Work out the finished part from the listing and answer in its coordinate system (mm). Face numbers are marked on the shaded views. A direction names the side the tool comes from. Coordinates: 2 decimals unless noted, no trailing zeros. Order: outer loops, then holes, each group sorted by start corner. A loop starts at its lowest first (then second) coordinate and runs counter-clockwise, first axis right, second up. Notation, with made-up numbers: (3.5, 0) -> (8.5, 0) arc R15 cw to (8.5, 27) -> close; hole circle Ø7 at (13.5, 57.5). An arc over 180 degrees is marked (long way). Use one line per item in the form item = value.
from build123d import *

# Parameters (mm, degrees)
F1_DEPTH = 20
F2_R     = 2.25
F3_DEPTH = 25
F6_DEPTH = 200
F8_DEPTH = 25


with BuildPart() as f1:
    # F0 (on Top) → F1 (new body)
    with BuildSketch(Plane.XY):
        with BuildLine():
            Line((-14.1666658925, 2), (-14.1666658925, 0.5))
            ThreePointArc((-14.1666658925, 0.5), (-14.0202192831, 0.1464466094), (-13.6666658925, 0))
            Line((-13.6666658925, 0), (55.3333341075, 0))
            ThreePointArc((55.3333341075, 0), (55.6868874981, 0.1464466094), (55.8333341075, 0.5))
            Line((55.8333341075, 0.5), (55.8333341075, 2))
            ThreePointArc((55.8333341075, 2), (55.6868874981, 2.3535533906), (55.3333341075, 2.5))
            Line((55.3333341075, 2.5), (42.8333341075, 2.5))
            ThreePointArc((42.8333341075, 2.5), (41.4191205451, 3.0857864376), (40.8333341075, 4.5))
            Line((40.8333341075, 4.5), (40.8333341075, 5))
            ThreePointArc((40.8333341075, 5), (39.3688680134, 8.5355339059), (35.8333341075, 10))
            Line((35.8333341075, 10), (5.8333341075, 10))
            ThreePointArc((5.8333341075, 10), (2.2978002016, 8.5355339059), (0.8333341075, 5))
            Line((0.8333341075, 5), (0.8333341075, 4.5))
            ThreePointArc((0.8333341075, 4.5), (0.2475476699, 3.0857864376), (-1.1666658925, 2.5))
            Line((-1.1666658925, 2.5), (-13.6666658925, 2.5))
            ThreePointArc((-13.6666658925, 2.5), (-14.0202192831, 2.3535533906), (-14.1666658925, 2))
        make_face()
        Polygon((3.2352578961, 6.25), (4.5342960018, 8.5), (7.1323722132, 8.5), (8.4314103188, 6.25), (7.1323722132, 4), (4.5342960018, 4), align=None, mode=Mode.SUBTRACT)
        Polygon((11.3126081653, 6.25), (12.3229711364, 8), (14.3436970786, 8), (15.3540600497, 6.25), (14.3436970786, 4.5), (12.3229711364, 4.5), align=None, mode=Mode.SUBTRACT)
        Polygon((19.1012832999, 6.25), (19.9673087037, 7.75), (21.6993595113, 7.75), (22.5653849151, 6.25), (21.6993595113, 4.75), (19.9673087037, 4.75), align=None, mode=Mode.SUBTRACT)
        Polygon((26.8899584345, 6.25), (27.611646271, 7.5), (29.055021944, 7.5), (29.7767097805, 6.25), (29.055021944, 5), (27.611646271, 5), align=None, mode=Mode.SUBTRACT)
        Polygon((34.6786335691, 6.25), (35.2559838383, 7.25), (36.4106843767, 7.25), (36.9880346459, 6.25), (36.4106843767, 5.25), (35.2559838383, 5.25), align=None, mode=Mode.SUBTRACT)
    extrude(amount=F1_DEPTH)

    # F2 (on face) → F3 (cut)
    with BuildSketch(Plane(origin=(0, 2.5, 0), x_dir=(-1, 0, 0), z_dir=(0, 1, 0))):
        with Locations((7.4166658925, 10)):
            Circle(F2_R)
        with Locations((-49.0833341075, 10)):
            Circle(F2_R)
    extrude(amount=-F3_DEPTH, mode=Mode.SUBTRACT)

    # F5 (on face) → F6 (cut)
    with BuildSketch(Plane(origin=(-14.1666658925, 0, 0), x_dir=(0, -1, 0), z_dir=(-1, 0, 0))):
        with BuildLine():
            Line((-2.5, 12.2343860567), (-2.5, 20))
            Line((-2.5, 20), (-10, 20))
            Line((-10, 20), (-10, 10))
            Line((-10, 10), (-4.5, 10))
            ThreePointArc((-4.5, 10), (-3.1579102698, 10.5129202042), (-2.5, 11.7902009315))
            Line((-2.5, 11.7902009315), (-2.5, 12.2343860567))
        make_face()
    extrude(amount=-F6_DEPTH, mode=Mode.SUBTRACT)

    # F7 (on face) → F8 (cut)
    with BuildSketch(Plane(origin=(0, 2.5, 0), x_dir=(-1, 0, 0), z_dir=(0, 1, 0))):
        with BuildLine():
            Line((-5.8333341075, 20), (-35.8333341075, 20))
            Line((-35.8333341075, 20), (-36.8333341075, 20))
            ThreePointArc((-36.8333341075, 20), (-36.1262273263, 19.7071067812), (-35.8333341075, 19))
            Line((-35.8333341075, 19), (-35.8333341075, 14.7902009315))
            ThreePointArc((-35.8333341075, 14.7902009315), (-34.9546544511, 12.668880588), (-32.8333341075, 11.7902009315))
            Line((-32.8333341075, 11.7902009315), (-8.8333341075, 11.7902009315))
            ThreePointArc((-8.8333341075, 11.7902009315), (-6.7120137639, 12.668880588), (-5.8333341075, 14.7902009315))
            Line((-5.8333341075, 14.7902009315), (-5.8333341075, 19))
            ThreePointArc((-5.8333341075, 19), (-5.5404408887, 19.7071067812), (-4.8333341075, 20))
            Line((-4.8333341075, 20), (-5.8333341075, 20))
        make_face()
    extrude(amount=-F8_DEPTH, mode=Mode.SUBTRACT)


solid = f1.part
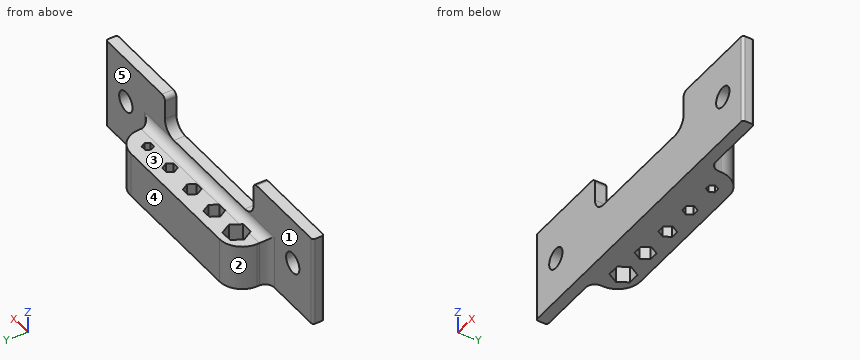
(1) Each of these flat-tipped pins is pushed along its axis until it touches: P1, Ø1.5, axis at y = 8.5, z = 5, coming from the -X side; P2, Ø1.5, axis at y = 4.5, z = 7.5, coming from the +X side; P3, Ø10, axis at x = 48.5, z = 11.5, coming from the +Y side. Where does it stop, or does it pass through?
Data:
P1 = 1.66
P2 = 40.98
P3 = 2.5
(2) Section B-B on z = 6 is taken. Count the separate pieces of the cut face and the enclosed holes in it, plus the area to 3 significant figures.
Data:
separate_pieces = 1
enclosed_holes = 5
area = 421 mm²
(3) Which of the six approach directions +Z, -Z, +X, -X, +Y, -Y give full straight-line access (tool end or side, diameter ignored) to the marked faces 1, 2, 3, 4 and 5?
Data:
face_1 = +Z, -X, +Y
face_2 = +Z, -Z, -X, +Y
face_3 = +Z, +X, -X, +Y
face_4 = +Z, -Z, +X, -X, +Y
face_5 = +Z, +X, +Y
(4) Straight lines are drawn through the part: line 1 along X through (y, z) = (2, 10); line 2 along Y through (x, z) = (12.5, 1.5); line 3 along X through (y, z) = (1, 17.5). For each, find the intervals that lie inside material, in ascending order.
Data:
line_1 = -14.17 to -9.67, -5.17 to 46.83, 51.33 to 55.83
line_2 = 0 to 4.5, 8 to 10
line_3 = -14.17 to 5.83, 35.83 to 55.83
(5) Section A-A on z = 16.25 is taken. Write down the section's boundary in (x, y).
Data:
outline = (-14.17, 0.5) arc R0.5 ccw to (-13.67, 0) -> (5.83, 0) -> (5.83, 2.5) -> (-13.67, 2.5) arc R0.5 ccw to (-14.17, 2) -> close; (35.83, 0) -> (55.33, 0) arc R0.5 ccw to (55.83, 0.5) -> (55.83, 2) arc R0.5 ccw to (55.33, 2.5) -> (35.83, 2.5) -> close
